```python
from build123d import *
from build123d.topology import SkipClean

# Parameters (mm, degrees)
SCHIZZO1_R                             = 30
SCHIZZO1_R_2                           = 3
ESTRUSIONE_ESTRUSIONE1_DEPTH           = 1.5
FORO_SVASATO_PER_VITE_M2_1_D           = 2.4
FORO_SVASATO_PER_VITE_M2_1_DEPTH       = 6
FORO_SVASATO_PER_VITE_M2_1_CSINK_D     = 4.4
FORO_SVASATO_PER_VITE_M2_1_CSINK_ANGLE = 90
FORO_SVASATO_PER_VITE_M2_1_TIP         = 0.721032743
SCHIZZO5_R                             = 4.5
ESTRUSIONE_ESTRUSIONE2_DEPTH           = 4
SCHIZZO9_R                             = 3
TAGLIO_ESTRUSIONE1_DEPTH               = 10


with BuildPart() as part:
    # Schizzo1 → Estrusione-Estrusione1 (new body)
    with BuildSketch(Plane.XY):
        Circle(SCHIZZO1_R)
        Circle(SCHIZZO1_R_2, mode=Mode.SUBTRACT)
    extrude(amount=ESTRUSIONE_ESTRUSIONE1_DEPTH)

    # Foro svasato per Vite M2-1
    with Locations(Plane(origin=(0, 0, 0), x_dir=(-1, 0, 0), z_dir=(0, 0, -1))):
        with Locations((0, -26), (-25, 3), (25, 3)):
            CounterSinkHole(FORO_SVASATO_PER_VITE_M2_1_D / 2, FORO_SVASATO_PER_VITE_M2_1_CSINK_D / 2, depth=FORO_SVASATO_PER_VITE_M2_1_DEPTH, counter_sink_angle=FORO_SVASATO_PER_VITE_M2_1_CSINK_ANGLE)
            with Locations((0, 0, -(FORO_SVASATO_PER_VITE_M2_1_DEPTH + FORO_SVASATO_PER_VITE_M2_1_TIP / 2))):  # 118° drill point
                Cone(0, FORO_SVASATO_PER_VITE_M2_1_D / 2, FORO_SVASATO_PER_VITE_M2_1_TIP, mode=Mode.SUBTRACT)

    # Schizzo5 → Estrusione-Estrusione2 (add)
    with BuildSketch(Plane(origin=(0, 0, 0), x_dir=(-1, 0, 0), z_dir=(0, 0, -1))):
        with Locations(Location((0, 0, 0), (0, 0, 180))):
            Circle(SCHIZZO5_R)
    extrude(amount=ESTRUSIONE_ESTRUSIONE2_DEPTH)

    # Schizzo9 → Taglio-Estrusione1 (cut)
    with SkipClean():  # the faces are left unmerged after this step: merging them gives an invalid solid
        with BuildSketch(Plane(origin=(0, 0, -4), x_dir=(-1, 0, 0), z_dir=(0, 0, -1))):
            Circle(SCHIZZO9_R)
        extrude(amount=-TAGLIO_ESTRUSIONE1_DEPTH, mode=Mode.SUBTRACT)


solid = part.part
```
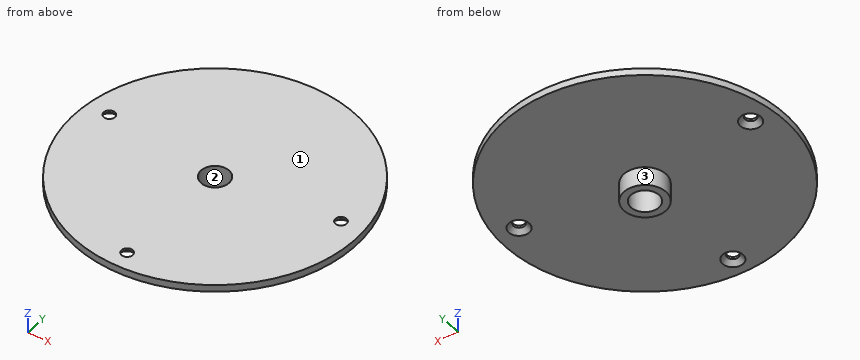
Geometry check sheet. Reference: the model listing, model coordinates, mm. Face numbers are marked on the shaded views. Round coordinates to 2 decimals unless told otherwise and drop trailing zeros. Loops run counter-clockwise (first coordinate to the right, second up) from the corner with the lowest first, then second, coordinate; pieces in that order, holes last. Notation, with made-up numbers: (-15.75, 3.25) -> (42.25, 3.25) arc R23 cw to (42.25, 15.25) -> close; hole circle Ø3 at (-37.75, -18). An arc over 180 degrees is marked (long way). Use a Markdown table: item, result.
(1) Go/stop test with flat-tipped pins: P1, Ø5.5, axis at x = 0, y = 0, coming from the -Z side; P2, Ø4, axis at x = 25, y = 3, coming from the +Z side; P3, Ø1.5, axis at y = -5.5, z = 0, coming from the -X side; P4, Ø1.5, axis at y = 1, z = -2, coming from the +X side. Record where each tip stops, or that it passes through.
Calculated:
| item | result |
|---|---|
| P1 | through |
| P2 | z = 1.5 |
| P3 | x = -29.62 |
| P4 | x = 4.49 |
(2) Sectioned sample at C-C (z = -2.9). Enter the section's corners in (x, y), then the cut area to 3 significant figures.
Calculated:
| item | result |
|---|---|
| outline | circle Ø9 at (0, 0); hole circle Ø6 at (0, 0) |
| area | 35.3 mm² |
(3) Sectioned sample at B-B (x = -25). Enter the section's corners in (y, z), then the cut area to 3 significant figures.
Calculated:
| item | result |
|---|---|
| outline | (-16.58, 0) -> (0.8, 0) -> (1.8, 1) -> (1.8, 1.5) -> (-16.58, 1.5) -> close; (4.2, 1) -> (5.2, 0) -> (16.58, 0) -> (16.58, 1.5) -> (4.2, 1.5) -> close |
| area | 45.1 mm² |
(4) Scan lines: probe 1 along Y at (x, z) = (0, 1.25); probe 2 along Y at (x, z) = (0, -2); probe 3 along Z at (x, y) = (-9, 26). Record each from-to range of solid material in increasing order.
Calculated:
| item | result |
|---|---|
| probe 1 | -30 to -27.2, -24.8 to -3, 3 to 30 |
| probe 2 | -4.5 to -3, 3 to 4.5 |
| probe 3 | 0 to 1.5 |
(5) Sectioned sample at A-A (x = 0). Enter the section's corners in (y, z).
Calculated:
| item | result |
|---|---|
| outline | (-30, 0) -> (-28.2, 0) -> (-27.2, 1) -> (-27.2, 1.5) -> (-30, 1.5) -> close; (-24.8, 1) -> (-23.8, 0) -> (-4.5, 0) -> (-4.5, -4) -> (-3, -4) -> (-3, 1.5) -> (-24.8, 1.5) -> close; (3, -4) -> (4.5, -4) -> (4.5, 0) -> (30, 0) -> (30, 1.5) -> (3, 1.5) -> close |
(6) Mould release check, pull along Y, two halves, no side actions. Record for the marked faces 1, 2 and 3: released by +Y, released by -Y, zero draft, split by the parting line, or undercut.
Calculated:
| item | result |
|---|---|
| face 1 | zero draft |
| face 2 | undercut |
| face 3 | split by the parting line |
(7) Sectioned sample at D-D (y = 26). Enter the section's corners in (x, z).
Calculated:
| item | result |
|---|---|
| outline | (-14.97, 0) -> (14.97, 0) -> (14.97, 1.5) -> (-14.97, 1.5) -> close |
